The listing builds one solid part. Answer for the finished solid, in the listing's coordinates (mm). A direction names the side the tool comes from. Coordinates: 2 decimals unless noted, no trailing zeros. Loops run counter-clockwise (first coordinate to the right, second up) from the corner with the lowest first, then second, coordinate; pieces in that order, holes last. Notation, with made-up numbers: M 79.25,45 L 88.25,45 A16 ccw 88.25,52 Z; hole C 64,23 d10. An arc over 180 degrees is marked long. Answer as CSV lines item,"result". Start each with the question number.
```python
from build123d import *

# Parameters (mm, degrees)
SKETCH3_W           = 11
SKETCH3_H           = 8.3
BOSS_EXTRUDE1_DEPTH = 2.4
SKETCH5_W           = 1
SKETCH5_H           = 1
CUT_EXTRUDE1_DEPTH  = 5
CHAMFER1_SIZE       = 0.5
SKETCH4_W           = 0.5
SKETCH4_H           = 0.35
BOSS_EXTRUDE2_DEPTH = 3


with BuildPart() as part:
    # Sketch3 → Boss-Extrude1 (new body)
    with BuildSketch(Plane.XY):
        Rectangle(SKETCH3_W, SKETCH3_H)
    extrude(amount=BOSS_EXTRUDE1_DEPTH)

    # Sketch5 → Cut-Extrude1 (cut)
    with BuildSketch(Plane(origin=(0, 4.15, 0), x_dir=(1, 0, 0), z_dir=(0, 1, 0))):
        with Locations((-3.81, -1.2)):
            Rectangle(SKETCH5_W, SKETCH5_H)
        with Locations((-1.27, -1.2)):
            Rectangle(SKETCH5_W, SKETCH5_H)
        with Locations((1.27, -1.2)):
            Rectangle(SKETCH5_W, SKETCH5_H)
        with Locations((3.81, -1.2)):
            Rectangle(SKETCH5_W, SKETCH5_H)
    extrude(amount=-CUT_EXTRUDE1_DEPTH, mode=Mode.SUBTRACT)

    # Chamfer1
    chamfer1_edges = [part.edges().sort_by_distance(p)[0] for p in [
        (-3.31, 4.15, 1.2),
        (-3.81, 4.15, 0.7),
        (-4.31, 4.15, 1.2),
        (-3.81, 4.15, 1.7),
        (-1.27, 4.15, 1.7),
        (-0.77, 4.15, 1.2),
        (-1.27, 4.15, 0.7),
        (-1.77, 4.15, 1.2),
        (1.27, 4.15, 1.7),
        (1.77, 4.15, 1.2),
        (1.27, 4.15, 0.7),
        (0.77, 4.15, 1.2),
        (3.81, 4.15, 1.7),
        (4.31, 4.15, 1.2),
        (3.81, 4.15, 0.7),
        (3.31, 4.15, 1.2),
    ]]
    chamfer(chamfer1_edges, length=CHAMFER1_SIZE)

    # Sketch4 → Boss-Extrude2 (add)
    with BuildSketch(Plane.XZ.offset(4.15)):
        with Locations((-1.27, 1.2)):
            Rectangle(SKETCH4_W, SKETCH4_H)
        with Locations((-3.81, 1.2)):
            Rectangle(SKETCH4_W, SKETCH4_H)
        with Locations((1.27, 1.2)):
            Rectangle(SKETCH4_W, SKETCH4_H)
        with Locations((3.81, 1.2)):
            Rectangle(SKETCH4_W, SKETCH4_H)
    extrude(amount=BOSS_EXTRUDE2_DEPTH)


solid = part.part
```
Item 1: Consider line 1 (X direction, y = 2.75, z = 0.8); line 2 (X direction, y = -5.5, z = 1.1); line 3 (Z direction, x = -1, y = 1.5). Determine where each line is inside the solid, lowest interval first.
Item 2: Section B-B on z = 0.35 is taken. Determine the outline of the cut face in (x, y), then the cut area to 3 significant figures.
Item 3: Section C-C on x = -4.5 is taken. Determine the outline of the cut face in (y, z).
Item 4: Section A-A on y = 2 is taken. Determine the outline of the cut face in (x, z), then the cut area to 3 significant figures.
Item 5: For faces 1 (the face through (0, 0, 2.4)), 2 (the face through (-1, 1, 0.7)), determine the directions among +Z, -Z, +X, -X, +Y, -Y from which every point of the face is accessible in a straight line to the end or side of a thin tool.
Item 6: Section D-D on y = -5 is taken. Determine the outline of the cut face in (x, z) (3 decimals).
Item 7: For a pull along Z with two mould halves and no side action, classify faces 3 (the face through (-1, 1, 1.7)), 4 (the face through (0, 0, 0)), 5 (the face through (0, -4.15, 1)), 6 (the face through (-1, -0.85, 1)) as pulls with the +Z half, pulls with the -Z half, needs draft (parallel to the pull), parting line crosses it, or undercut.
Item 8: This flat-tipped pin is pushed along its axis until it touches: P1, Ø0.5, axis at x = 4, z = 1.5, coming from the +Y side. Where does it stop, or does it pass through?
Results are:
1,line 1,"-5.5 to -4.31, -3.31 to -1.77, -0.77 to 0.77, 1.77 to 3.31, 4.31 to 5.5"
1,line 2,"-4.06 to -3.56, -1.52 to -1.02, 1.02 to 1.52, 3.56 to 4.06"
1,line 3,"0 to 0.7, 1.7 to 2.4"
2,outline,"M -5.5,-4.15 L 5.5,-4.15 L 5.5,4.15 L 4.81,4.15 L 4.66,4 L 2.96,4 L 2.81,4.15 L 2.27,4.15 L 2.12,4 L 0.42,4 L 0.27,4.15 L -0.27,4.15 L -0.42,4 L -2.12,4 L -2.27,4.15 L -2.81,4.15 L -2.96,4 L -4.66,4 L -4.81,4.15 L -5.5,4.15 Z"
2,area,"90.2 mm²"
3,outline,"M -4.15,0 L 4.15,0 L 4.15,0.2 L 3.84,0.51 L 3.84,1.89 L 4.15,2.2 L 4.15,2.4 L -4.15,2.4 Z"
4,outline,"M -5.5,0 L 5.5,0 L 5.5,2.4 L -5.5,2.4 Z; hole M -4.31,0.7 L -3.31,0.7 L -3.31,1.7 L -4.31,1.7 Z; hole M -1.77,0.7 L -0.77,0.7 L -0.77,1.7 L -1.77,1.7 Z; hole M 0.77,0.7 L 1.77,0.7 L 1.77,1.7 L 0.77,1.7 Z; hole M 3.31,0.7 L 4.31,0.7 L 4.31,1.7 L 3.31,1.7 Z"
4,area,"22.4 mm²"
5,face 1,"+Z, +X, -X, +Y, -Y"
5,face 2,"+Y"
6,outline,"M -4.06,1.025 L -3.56,1.025 L -3.56,1.375 L -4.06,1.375 Z; M -1.52,1.025 L -1.02,1.025 L -1.02,1.375 L -1.52,1.375 Z; M 1.02,1.025 L 1.52,1.025 L 1.52,1.375 L 1.02,1.375 Z; M 3.56,1.025 L 4.06,1.025 L 4.06,1.375 L 3.56,1.375 Z"
7,face 3,"undercut"
7,face 4,"pulls with the -Z half"
7,face 5,"needs draft"
7,face 6,"undercut"
8,P1,"y = 3.7"
